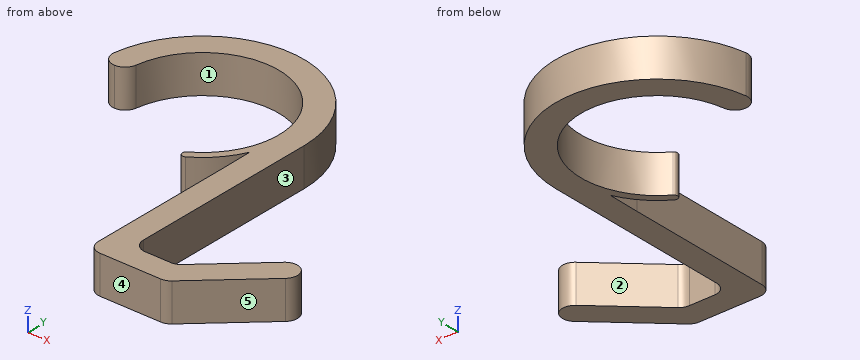
```python
from build123d import *

# Parameters (mm, degrees)
F1_DEPTH    = 15
F2_T1_DEPTH = 15
F2_T3_DEPTH = 38.2179411812
F2_T5_DEPTH = 43.6185312436
F2_T7_DEPTH = 40
F2_T9_DEPTH = 24.832214185
F3_R        = 1.49999


# Not quite as in the source:
# - a fillet or chamfer that OpenCascade refuses, or shapes differently, is made with other operations: its cross-section is extruded or revolved along the edge and cut away or added
# - a fillet or chamfer is up to 0.001 mm smaller than in the source, because OpenCascade refuses the exact size


with BuildPart() as f1:
    # F0 (on Top) → F1 (new body)
    with BuildSketch(Plane.XY):
        with BuildLine():
            ThreePointArc((-30.25, 0), (15.4242466579, 26.0222042694), (14.5205861182, -26.5370510567))
            Line((14.5205861182, -26.5370510567), (15.9606442456, -29.1688247152))
            ThreePointArc((15.9606442456, -29.1688247152), (24.4038188383, -22.5835366164), (30.3161764706, -13.6562053369))
            Line((30.3161764706, -13.6562053369), (30.4329268293, -26.3419715398))
            Line((30.4329268293, -26.3419715398), (30.4329268293, -89.5091558098))
            Line((30.4329268293, -89.5091558098), (61.4327350343, -89.5091558098))
            Line((61.4327350343, -89.5091558098), (91.6112407267, -61.4279471198))
            Line((91.6112407267, -61.4279471198), (84.9590376288, -54.2789119314))
            Line((84.9590376288, -54.2789119314), (57.316922531, -80))
            Line((57.316922531, -80), (40.25, -80))
            Line((40.25, -80), (40.25, 0))
            ThreePointArc((40.25, 0), (0, 40.25), (-40.25, 0))
            Line((-40.25, 0), (-30.25, 0))
        make_face()
    extrude(amount=F1_DEPTH)

    # F2: fillet of radius 5 on 8 edges, made by hand

    # F2_s2 → F2_t1 (join)
    with BuildSketch(Plane.XY):
        with BuildLine():
            ThreePointArc((45.25, -80), (41.7144660941, -78.5355339059), (40.25, -75))
            Line((40.25, -75), (40.25, -80))
            Line((40.25, -80), (45.25, -80))
        make_face()
        with BuildLine():
            ThreePointArc((58.7565312825, -78.6604388503), (57.1804804794, -79.6530739437), (55.350479694, -80))
            Line((55.350479694, -80), (57.316922531, -80))
            Line((57.316922531, -80), (58.7565312825, -78.6604388503))
        make_face()
    extrude(amount=F2_T1_DEPTH)

    # F2_s4 → F2_t3 (cut)
    with BuildSketch(Plane.XY.offset(-11.6089705906)):
        with BuildLine():
            ThreePointArc((-29.9441430963, 4.2907801418), (-31.6183858983, 1.2220310158), (-34.8935882362, 0))
            Line((-34.8935882362, 0), (-30.25, 0))
            ThreePointArc((-30.25, 0), (-30.1734388881, 2.1508337146), (-29.9441430963, 4.2907801418))
        make_face()
    extrude(amount=F2_T3_DEPTH, mode=Mode.SUBTRACT)

    # F2_s6 → F2_t5 (cut)
    with BuildSketch(Plane.XY.offset(-14.3092656218)):
        with BuildLine():
            ThreePointArc((-34.8935882362, 0), (-38.6715572204, 1.724797662), (-39.8430333761, 5.7092198582))
            ThreePointArc((-39.8430333761, 5.7092198582), (-40.1481294296, 2.8618531244), (-40.25, 0))
            Line((-40.25, 0), (-34.8935882362, 0))
        make_face()
    extrude(amount=F2_T5_DEPTH, mode=Mode.SUBTRACT)

    # F2_s8 → F2_t7 (cut)
    with BuildSketch(Plane.XY.offset(-12.5)):
        with BuildLine():
            ThreePointArc((88.3650892173, -57.9393507817), (84.8845293249, -56.3486390617), (81.2985987785, -57.6849635199))
            Line((81.2985987785, -57.6849635199), (84.9590376288, -54.2789119314))
            Line((84.9590376288, -54.2789119314), (88.3650892173, -57.9393507817))
        make_face()
        with BuildLine():
            ThreePointArc((87.9508018764, -64.8339987083), (89.5415135964, -61.3534388159), (88.2051891382, -57.7675082695))
            Line((88.2051891382, -57.7675082695), (91.6112407267, -61.4279471198))
            Line((91.6112407267, -61.4279471198), (87.9508018764, -64.8339987083))
        make_face()
        with BuildLine():
            ThreePointArc((30.4329268293, -84.5091558098), (31.8973929233, -88.0446897157), (35.4329268293, -89.5091558098))
            Line((35.4329268293, -89.5091558098), (30.4329268293, -89.5091558098))
            Line((30.4329268293, -89.5091558098), (30.4329268293, -84.5091558098))
        make_face()
    extrude(amount=F2_T7_DEPTH, mode=Mode.SUBTRACT)

    # F2_s10 → F2_t9 (cut)
    with BuildSketch(Plane.XY.offset(-4.9161070925)):
        with BuildLine():
            ThreePointArc((59.4662921973, -89.5091558098), (61.2962929826, -89.1622297535), (62.8723437858, -88.1695946601))
            Line((62.8723437858, -88.1695946601), (61.4327350343, -89.5091558098))
            Line((61.4327350343, -89.5091558098), (59.4662921973, -89.5091558098))
        make_face()
    extrude(amount=F2_T9_DEPTH, mode=Mode.SUBTRACT)

    # F3 (radius 1.5 in the source; OpenCascade refuses exactly that, so slightly less here)
    f3_edges = [f1.edges().sort_by_distance(p)[0] for p in [
        (14.520586, -26.537051, 7.5),
        (15.960644, -29.168825, 7.5),
    ]]
    fillet(f3_edges, radius=F3_R)


solid = f1.part
```
Read the model definition and answer for the solid it produces. Units are mm, in the model's axes. Face numbers are marked on the shaded views. A direction names the side the tool comes from. Coordinates: 2 decimals unless noted, no trailing zeros. Loops run counter-clockwise (first coordinate to the right, second up) from the corner with the lowest first, then second, coordinate; pieces in that order, holes last.
(1) The mould has two halves that part along X. Classify the marked faces 3, 4 and 5: released by +X, released by -X, zero draft, split by the parting line, or undercut.
Solution:
face 3: undercut
face 4: zero draft
face 5: released by +X
(2) Consider line 1 along X through (y, z) = (27, 1.5); line 2 along Y through (x, z) = (0, 11.75); line 3 along X through (y, z) = (-44.5, 10.5). Determine where each line is inside the solid, lowest interval first.
Solution:
line 1: x = -29.85 to -13.64, 13.64 to 29.85
line 2: y = 30.25 to 40.25
line 3: x = 30.43 to 40.25
(3) A tool of negligible diameter and unlimited length cuts with its end or side. For the marked faces 1 and 2, from which of +Z, -Z, +X, -X, +Y, -Y can it reach the whole face along a straight path? Write none if from no direction.
Solution:
face 1: +Z, -Z
face 2: +Z, -Z, +Y
(4) The part is cut by section A-A (y = 12.5). Determine the outline of the cut face in (x, z), and give its area (3 significant figures).
Solution:
outline: (-38.26, 0) - (-27.55, 0) - (-27.55, 15) - (-38.26, 15) - close; (27.55, 0) - (38.26, 0) - (38.26, 15) - (27.55, 15) - close
area: 321 mm2
(5) Flat-ended cylindrical pins translate along their axes: pin 1 Ø6 at (x, z) = (67, 4.5) entering from +Y; pin 2 Ø4 at (y, z) = (-64, 6) entering from -X; pin 3 Ø1 at (x, z) = (-11.5, 13) entering from -Y. Find the tip coordinate at first contact, or state that the pin passes through.
Solution:
pin 1: stops at y = -68.2
pin 2: stops at x = 30.43
pin 3: stops at y = 27.77
(6) The part is cut by section C-C (x = 0). Determine the outline of the cut face in (y, z), and give its area (3 significant figures).
Solution:
outline: (30.25, 0) - (40.25, 0) - (40.25, 15) - (30.25, 15) - close
area: 150 mm2
(7) The part is cut by section D-D (y = -24). Determine the outline of the cut face in (x, z), and give its area (3 significant figures).
Solution:
outline: (18.41, 0) - (23.01, 0) - (23.01, 15) - (18.41, 15) - close; (30.41, 0) - (40.25, 0) - (40.25, 15) - (30.41, 15) - close
area: 217 mm2
